Check sheet for the modelled part. Datum: model origin and axes. Units: mm. Face numbers are marked on the shaded views. A direction names the side the tool comes from. Coordinates: 2 decimals unless noted, no trailing zeros. Order: outer loops, then holes, each group sorted by start corner. A loop starts at its lowest first (then second) coordinate and runs counter-clockwise, first axis right, second up.
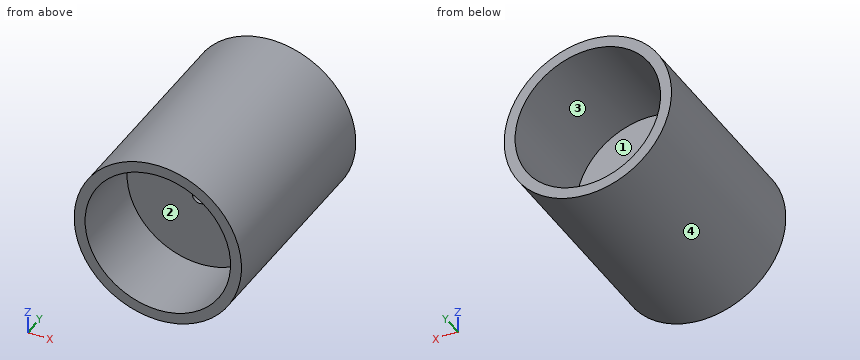
from build123d import *

# Parameters (mm, degrees)
SKETCH1_R           = 23
BOSS_EXTRUDE1_DEPTH = 60
SKETCH2_R           = 20
CUT_EXTRUDE1_DEPTH  = 22
CUT_EXTRUDE2_START  = -32
SKETCH5_R           = 20
CUT_EXTRUDE2_DEPTH  = 32
SKETCH4_R           = 2
CUT_EXTRUDE3_DEPTH  = 40


with BuildPart() as part:
    # Sketch1 → Boss-Extrude1 (new body)
    with BuildSketch(Plane(origin=(0, 0, 0), x_dir=(1, 0, 0), z_dir=(0, 1, 0))):
        with Locations(Location((0, 0, 0), (0, 0, 270))):
            Circle(SKETCH1_R)
    extrude(amount=BOSS_EXTRUDE1_DEPTH)

    # Sketch2 → Cut-Extrude1 (cut)
    with BuildSketch(Plane.XZ):
        with Locations(Location((0, 0, 0), (0, 0, 270))):
            Circle(SKETCH2_R)
    extrude(amount=-CUT_EXTRUDE1_DEPTH, mode=Mode.SUBTRACT)

    # Sketch5 → Cut-Extrude2 (cut)
    with BuildSketch(Plane(origin=(0, 60, 0), x_dir=(1, 0, 0), z_dir=(0, 1, 0)).offset(CUT_EXTRUDE2_START)):
        with Locations(Location((0, 0, 0), (0, 0, 90))):
            Circle(SKETCH5_R)
    extrude(amount=CUT_EXTRUDE2_DEPTH, mode=Mode.SUBTRACT)

    # Sketch4 → Cut-Extrude3 (cut)
    with BuildSketch(Plane.XZ.offset(-22)):
        with Locations(Location((0, 0, 0), (0, 0, 270))):
            Circle(SKETCH4_R)
    extrude(amount=-CUT_EXTRUDE3_DEPTH, mode=Mode.SUBTRACT)


solid = part.part
(1) Cross-section at A-A (z = 0). Enter the section's corners in (x, y), and give its area (3 significant figures).
Filled in:
outline: (-23, 0) - (-20, 0) - (-20, 22) - (-2, 22) - (-2, 28) - (-20, 28) - (-20, 60) - (-23, 60) - close; (2, 22) - (20, 22) - (20, 0) - (23, 0) - (23, 60) - (20, 60) - (20, 28) - (2, 28) - close
area: 576 mm2
(2) Go/stop test with flat-tipped pins: P1, Ø5, axis at y = 45.5, z = 1, coming from the -X side; P2, Ø2, axis at x = -12.5, y = 37.5, coming from the -Z side; P3, Ø12, axis at x = 11, z = 1, coming from the +Y side; P4, Ø3.5, axis at x = 0, z = 0, coming from the -Y side. Record where each tip stops, or that it passes through.
Filled in:
P1: stops at x = -23
P2: stops at z = -19.92
P3: stops at y = 28
P4: passes through
(3) Cross-section at C-C (y = 54.5). Enter the section's corners in (x, z), and give its area (3 significant figures).
Filled in:
outline: circle Ø46 at (0, 0); hole circle Ø40 at (0, 0)
area: 405 mm2
(4) Thickness scan on probe 1 along X at (y, z) = (38.5, 0); probe 2 along Y at (x, z) = (-16.5, 7); probe 3 along X at (y, z) = (29, 7.5). Record the ranges inside material, lowest first.
Filled in:
probe 1: x = -23 to -20, 20 to 23
probe 2: y = 22 to 28
probe 3: x = -21.74 to -18.54, 18.54 to 21.74
(5) Release check for a two-part mould opening along Z. For the marked faces 3 and 4 record: +Z half, -Z half, draft (parallel to the pull), parting line (faces both ways), or undercut.
Filled in:
face 3: undercut
face 4: parting line
(6) Cross-section at B-B (x = 0). Enter the section's corners in (y, z).
Filled in:
outline: (0, -23) - (60, -23) - (60, -20) - (28, -20) - (28, -2) - (22, -2) - (22, -20) - (0, -20) - close; (0, 20) - (22, 20) - (22, 2) - (28, 2) - (28, 20) - (60, 20) - (60, 23) - (0, 23) - close
(7) Cross-section at D-D (x = 6). Enter the section's corners in (y, z).
Filled in:
outline: (0, -22.2) - (60, -22.2) - (60, -19.08) - (28, -19.08) - (28, 19.08) - (60, 19.08) - (60, 22.2) - (0, 22.2) - (0, 19.08) - (22, 19.08) - (22, -19.08) - (0, -19.08) - close
(8) Tool access check on the marked faces 1 and 2. Record the directions out of +Z, -Z, +X, -X, +Y, -Y that give a thin tool (end or side, any length) a straight path to the whole face; none if there is none.
Filled in:
face 1: +Y
face 2: -Y
